Here's how the part is built. I have some questions about the finished solid (model axes, mm). Round coordinates to 2 decimals unless told otherwise and drop trailing zeros. Write each loop counter-clockwise with the first axis right and the second up, starting at its lowest first coordinate (ties: lowest second). Pieces come first, ordered by that corner, then holes. Notation, with made-up numbers: (42, 48) - (52, 48) arc R24 cw to (52, 67) - close; hole circle Ø3 at (34, -21.75). An arc over 180 degrees is marked (long way). One line per item, written item: value. Start each with the question number.
Item 1: Imagine slicing it at D-D, the plane x = 15.5. Please give me the cut outline in (y, z) (3 decimals).
Item 2: If I drill on line 1 (X direction, y = -1.75, z = 0); line 2 (Z direction, x = -27.5, y = -2); line 3 (X direction, y = -1.65, z = -7), over which ranges is the centre line in solid material (lowest first)?
Item 3: Imagine slicing it at B-B, the plane z = 0. Count the separate pieces of the cut face and the enclosed holes in it, then the cut area to 3 significant figures.
Item 4: For P1, Ø5, axis at x = 36.51, z = 22.22, coming from the -Y side, with a flat end and sliding along its axis, tell me the tip position at first contact or that it passes through.
Item 5: Imagine slicing it at A-A, the plane x = 0. Please give me the cut outline in (y, z) (3 decimals), then the cut area to 3 significant figures.
Item 6: Thinking about a two-plate mould opening in X: for faces 1 (the face through (5, 0, 6)), 2 (the face through (40.953, -1.565, -14.064)), 3 (the face through (35.3, -1.57, 25.16)), which applies, released by +X, released by -X, zero draft, split by the parting line, or undercut?
```python
from build123d import *

# Parameters (mm, degrees)
BASE_FLANGE1_DEPTH = 3.175
SKETCH6_R          = 3.175
SKETCH6_R_2        = 6
SKETCH6_R_3        = 1.25
CUT_EXTRUDE1_DEPTH = 52.612064057


# Sheet-metal steps are written as plain solids
with BuildPart() as part:
    # Sketch1 → Base-Flange1 (new body)
    with BuildSketch(Plane(origin=(0, 0, 0), x_dir=(1, 0, 0), z_dir=(0, 1, 0))):
        with BuildLine():
            Line((36.5125, -28.575), (-26.9875, -28.575))
            ThreePointArc((-26.9875, -28.575), (-31.477628061, -26.715128061), (-33.3375, -22.225))
            Line((-33.3375, -22.225), (-33.3375, 9.525))
            ThreePointArc((-33.3375, 9.525), (-31.477628061, 14.015128061), (-26.9875, 15.875))
            Line((-26.9875, 15.875), (36.5125, 15.875))
            ThreePointArc((36.5125, 15.875), (41.002628061, 14.015128061), (42.8625, 9.525))
            Line((42.8625, 9.525), (42.8625, -22.225))
            ThreePointArc((42.8625, -22.225), (41.002628061, -26.715128061), (36.5125, -28.575))
        make_face()
    extrude(amount=-BASE_FLANGE1_DEPTH)

    # Sketch6 → Cut-Extrude1 (cut, through all)
    with BuildSketch(Plane(origin=(0, 0, 0), x_dir=(1, 0, 0), z_dir=(0, 1, 0))):
        with Locations(Location((-26.9875, 9.525, 0), (0, 0, 270))):
            Circle(SKETCH6_R)
        with Locations(Location((-26.9875, -22.225, 0), (0, 0, 270))):
            Circle(SKETCH6_R)
        with Locations(Location((36.5125, 9.525, 0), (0, 0, 270))):
            Circle(SKETCH6_R)
        with Locations(Location((36.5125, -22.225, 0), (0, 0, 270))):
            Circle(SKETCH6_R)
        with Locations(Location((0, 7, 0), (0, 0, 270))):
            Circle(SKETCH6_R_2)
        with Locations(Location((-15.5, 0, 0), (0, 0, 270))):
            Circle(SKETCH6_R_3)
        with Locations(Location((15.5, 0, 0), (0, 0, 270))):
            Circle(SKETCH6_R_3)
    extrude(amount=-CUT_EXTRUDE1_DEPTH, mode=Mode.SUBTRACT)


solid = part.part
```
Values follow:
1. outline: (-3.175, -15.875) - (0, -15.875) - (0, -1.25) - (-3.175, -1.25) - close; (-3.175, 1.25) - (0, 1.25) - (0, 28.575) - (-3.175, 28.575) - close
2. line 1: x = -33.34 to -16.75, -14.25 to 14.25, 16.75 to 42.86
2. line 2: z = -15.85 to -12.66, -6.39 to 19.09, 25.36 to 28.55
2. line 3: x = -33.34 to -28.91, -25.06 to -6, 6 to 34.59, 38.44 to 42.86
3. separate pieces: 3
3. enclosed holes: 0
3. area: 226 mm^2
4. P1: passes through
5. outline: (-3.175, -15.875) - (0, -15.875) - (0, -13) - (-3.175, -13) - close; (-3.175, -1) - (0, -1) - (0, 28.575) - (-3.175, 28.575) - close
5. area: 103 mm^2
6. face 1: zero draft
6. face 2: released by +X
6. face 3: undercut
